Here's how the part is built. I have some questions about the finished solid (model axes, mm). A direction names the side the tool comes from. Give positions to 0.01 mm unless a question says otherwise; leave off trailing zeros. Write each loop counter-clockwise with the first axis right and the second up, starting at its lowest first coordinate (ties: lowest second). Pieces come first, ordered by that corner, then holes. Notation, with made-up numbers: (-4.75, -8) - (36.25, -8) arc R26 ccw to (36.25, 20) - close; hole circle Ø1 at (43, -27). An arc over 180 degrees is marked (long way). Use a Markdown table: item, result.
```python
from build123d import *

# Parameters (mm, degrees)
F1_DEPTH  = 6.35
F2_DEPTH  = 1.27
F3_W      = 1.27
F3_H      = 85.6234
F4_DEPTH  = 54.0004
F5_DEPTH  = 1.27
F6_W      = 1.27
F6_H      = 85.6234
F7_DEPTH  = 54.0004
F8_R      = 4.44499
F9_DEPTH  = 0.635
F10_DEPTH = 0.635


# Not quite as in the source:
# - a fillet or chamfer is up to 0.001 mm smaller than in the source, because OpenCascade refuses the exact size


with BuildPart() as f1:
    # F0 (on Front) → F1 (new body)
    with BuildSketch(Plane.XZ):
        Polygon((54.0004, 0), (0, 0), (0, 85.6234), (-5.08, 85.6234), (-5.08, 0), (-5.08, -5.08), (0, -5.08), (54.0004, -5.08), (59.0804, -5.08), (59.0804, 0), (59.0804, 85.6234), (54.0004, 85.6234), align=None)
    extrude(amount=F1_DEPTH)

    # F2 (add): a face of the model
    f2_faces = [f1.faces().sort_by_distance(p)[0] for p in [
        (27.0002, -6.35, -3.9689795817),
    ]]
    extrude(f2_faces, amount=F2_DEPTH)

    # F3 (on face) → F4 (join)
    with BuildSketch(Plane(origin=(54.0004, 0, 0), x_dir=(0, -1, 0), z_dir=(-1, 0, 0))):
        with Locations((6.985, 42.8117)):
            Rectangle(F3_W, F3_H)
    extrude(amount=F4_DEPTH)

    # F5 (add): a face of the model
    f5_faces = [f1.faces().sort_by_distance(p)[0] for p in [
        (27.0002, 0, -3.9689795817),
    ]]
    extrude(f5_faces, amount=F5_DEPTH)

    # F6 (on face) → F7 (join)
    with BuildSketch(Plane(origin=(54.0004, 0, 0), x_dir=(0, -1, 0), z_dir=(-1, 0, 0))):
        with Locations((-0.635, 42.8117)):
            Rectangle(F6_W, F6_H)
    extrude(amount=F7_DEPTH)

    # F8 (radius 4.445 in the source; OpenCascade refuses exactly that, so slightly less here)
    f8_edges = [f1.edges().sort_by_distance(p)[0] for p in [
        (-5.08, -7.62, 40.2717),
        (-5.08, 1.27, 40.2717),
        (59.0804, 1.27, 40.2717),
        (59.0804, -7.62, 40.2717),
        (-5.08, -3.175, -5.08),
        (27.0002, 1.27, -5.08),
        (27.0002, -7.62, -5.08),
        (59.0804, -3.175, -5.08),
    ]]
    fillet(f8_edges, radius=F8_R)

    # F9 (add): a face of the model
    f9_faces = [f1.faces().sort_by_distance(p)[0] for p in [
        (27.0002, 0, 42.8117),
    ]]
    extrude(f9_faces, amount=F9_DEPTH)

    # F10 (add): a face of the model
    f10_faces = [f1.faces().sort_by_distance(p)[0] for p in [
        (27.0002, -6.35, 42.8117),
    ]]
    extrude(f10_faces, amount=F10_DEPTH)


solid = f1.part
```
Item 1: For faces 1 (the flat face through (27, -6, 85.623)), 2 (the flat face through (27, -0.635, 42)), which set-ups out of +Z, -Z, +X, -X, +Y, -Y let a thin tool reach every point of the face, with its end or its side?
Values:
| item | result |
|---|---|
| face 1 | +Z, +X, -X, +Y, -Y |
| face 2 | +Z |
Item 2: If we section it at C-C, the plane y = -4.5: Write out the boundary of the cut face in (x, z) (3 decimals).
Values:
| item | result |
|---|---|
| outline | (-4.878, -0.635) arc R4.243 ccw to (-0.635, -4.878) - (54.635, -4.878) arc R4.243 ccw to (58.878, -0.635) - (58.878, 85.623) - (54, 85.623) - (54, 0) - (0, 0) - (0, 85.623) - (-4.878, 85.623) - close |
Item 3: Will these pins go through, and if not, where does the flat tip stop? pin 1 Ø3 at (y, z) = (-0.5, 19) entering from +X; pin 2 Ø1 at (x, y) = (34.5, -4.5) entering from +Z.
Values:
| item | result |
|---|---|
| pin 1 | stops at x = 58.92 |
| pin 2 | stops at z = 0 |
Item 4: I need wall thicknesses on line 1 along Y through (x, z) = (29, 57) (3 decimals); line 2 along X through (y, z) = (-2.5, 7); line 3 along X through (y, z) = (-4.75, 35). Which ranges of each line are inside material? Lowest first, please. Write a range as [from, to].
Values:
| item | result |
|---|---|
| line 1 | y = [-7.62, -5.715], [-0.635, 1.27] |
| line 2 | x = [-5.03, 0], [54, 59.03] |
| line 3 | x = [-4.79, 0], [54, 58.79] |
Item 5: Thinking about a two-plate mould opening in Y: for faces 3 (the flat face through (27, 1.27, 42)), 4 (the flat face through (54, -3, 43)), 5 (the flat face through (27, -7.62, 42)), which applies, +Y half, -Y half, draft (parallel to the pull), parting line (faces both ways), or undercut?
Values:
| item | result |
|---|---|
| face 3 | +Y half |
| face 4 | undercut |
| face 5 | -Y half |
